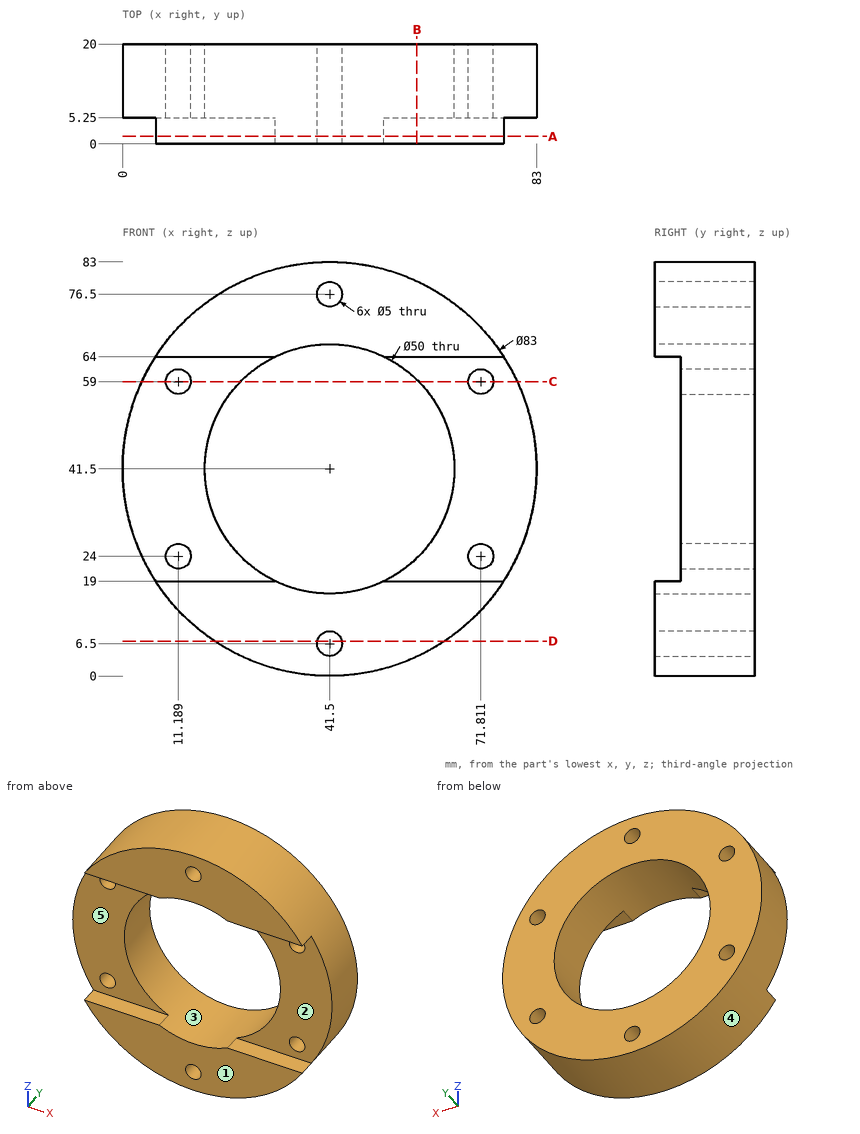
Input: dimensioned drawing with shaded views. Units: mm. Origin: part minimum x, y, z. A direction names the side the tool comes from. Round coordinates to 2 decimals unless told otherwise and drop trailing zeros. Order: outer loops, then holes, each group sorted by start corner. A loop starts at its lowest first (then second) coordinate and runs counter-clockwise, first axis right, second up. Notation, with made-up numbers: (59, 66.25) - (94, 66.25) arc R32 cw to (94, 101.25) - close; hole circle Ø11 at (57, 79.25). An arc over 180 degrees is marked (long way). Write item = value, one per line. Start each with the question number.
Q1. Access query for the marked faces 1 and 2. Directions: +Z, -Z, +X, -X, +Y, -Y. A direction counts if a zero-diameter tool reaches every point of the face in a straight line with its end or side. Return the directions, or none.
Q2. Cut plane B-B on x = 59. Return the cut outline in (y, z).
Q3. Cut plane D-D on z = 7. Return the cut outline in (x, y) (1 decimal).
Q4. Pin query (flat end, axial travel): pin 1 (2.5 mm diameter, centred on x = 23.5, y = 3, fed in from -Z); pin 2 (3 mm diameter, centred on x = 41.5, z = 76.5, fed in from -Y); pin 3 (1.5 mm diameter, centred on y = 2.5, z = 11.5, fed in from -X); pin 4 (12 mm diameter, centred on x = 67, z = 12, fed in from -Y). Return the tip coordinate at first contact, or that it passes through.
Q5. Ray query, line 1 (X direction, y = 11, z = 42.5); line 2 (Z direction, x = 9.5, y = 8) (1 decimal); line 3 (X direction, y = 12.5, z = 24). Return the intervals inside material, ascending. Write a range as from..to.
Q6. Cut plane A-A on y = 1.5. Return the cut outline in (x, z), and give its area (4 significant figures).
Q7. Pull-direction query (X, two-part tool) for the marked faces 3, 4 and 5; classes: +X half, -X half, draft (parallel to the pull), parting line (faces both ways), or undercut.
Q8. Cut plane C-C on z = 59. Return the cut outline in (x, y).
Outcome:
q1.face_1 = +Z, -Z, +X, -X, -Y
q1.face_2 = +X, -X, -Y
q2.outline = (0, 3.87) - (20, 3.87) - (20, 23.65) - (5.25, 23.65) - (5.25, 19) - (0, 19) - close; (0, 64) - (5.25, 64) - (5.25, 59.35) - (20, 59.35) - (20, 79.13) - (0, 79.13) - close
q3.outline = (18.4, 0) - (39.1, 0) - (39.1, 20) - (18.4, 20) - close; (43.9, 0) - (64.6, 0) - (64.6, 20) - (43.9, 20) - close
q4.pin_1 = 3.53
q4.pin_2 = through
q4.pin_3 = 12.06
q4.pin_4 = 0
q5.line_1 = 0.01..16.52, 66.48..82.99
q5.line_2 = 15.1..22.2, 25.8..57.2, 60.8..67.9
q5.line_3 = 3.87..8.69, 13.69..23.65, 59.35..69.31, 74.31..79.13
q6.outline = (6.63, 19) arc R41.5 ccw to (76.37, 19) - (52.4, 19) arc R25 cw to (30.6, 19) - close; (6.63, 64) - (30.6, 64) arc R25 cw to (52.4, 64) - (76.37, 64) arc R41.5 ccw to start; hole circle Ø5 at (41.5, 6.5); hole circle Ø5 at (41.5, 76.5)
q6.area = 1,755 mm^2
q7.face_3 = undercut
q7.face_4 = parting line
q7.face_5 = draft
q8.outline = (3.87, 5.25) - (8.69, 5.25) - (8.69, 20) - (3.87, 20) - close; (13.69, 5.25) - (23.65, 5.25) - (23.65, 20) - (13.69, 20) - close; (59.35, 5.25) - (69.31, 5.25) - (69.31, 20) - (59.35, 20) - close; (74.31, 5.25) - (79.13, 5.25) - (79.13, 20) - (74.31, 20) - close
